Input: dimensioned drawing with shaded views. Units: mm. Origin: part minimum x, y, z. A direction names the side the tool comes from. Coordinates: 2 decimals unless noted, no trailing zeros. Loops run counter-clockwise (first coordinate to the right, second up) from the corner with the lowest first, then second, coordinate; pieces in that order, holes last.
Item 1: Section B-B on x = 49.5. Return loops of the section in (y, z).
Item 2: Contact query for flat-ended pins moving along their axis: P1, Ø12, axis at y = 18, z = 17.5, coming from the -X side; P2, Ø4, axis at x = 32.5, y = 26, coming from the +Z side; P3, Ø6, axis at x = 21.5, y = 37, coming from the +Z side; P4, Ø1, axis at y = 39.5, z = 49.5, coming from the +X side. Output: stop coordinate, or through.
Item 3: Section D-D on z = 40. Return loops of the section in (x, y), and give its area (3 significant figures).
Item 4: Ray query, line 1 along Z through (x, y) = (5.5, 25); line 2 along X through (y, z) = (33, 19); line 3 along Z through (x, y) = (39, 38.5). Return the intervals inside material, ascending.
Item 5: Section A-A on z = 56. Return loops of the section in (x, y), and give its area (3 significant figures).
Item 6: Pull-direction query (Z, two-part tool) for the marked faces 4, 5, 6 and 7; classes: released by +Z, released by -Z, zero draft, split by the parting line, or undercut.
Item 7: Reachability of the marked faces 1, 2 and 3 from +Z, -Z, +X, -X, +Y, -Y: full face, straight path, thin tool, end or side. Return the list, or none.
Item 8: Section C-C on y = 21. Return loops of the section in (x, z).
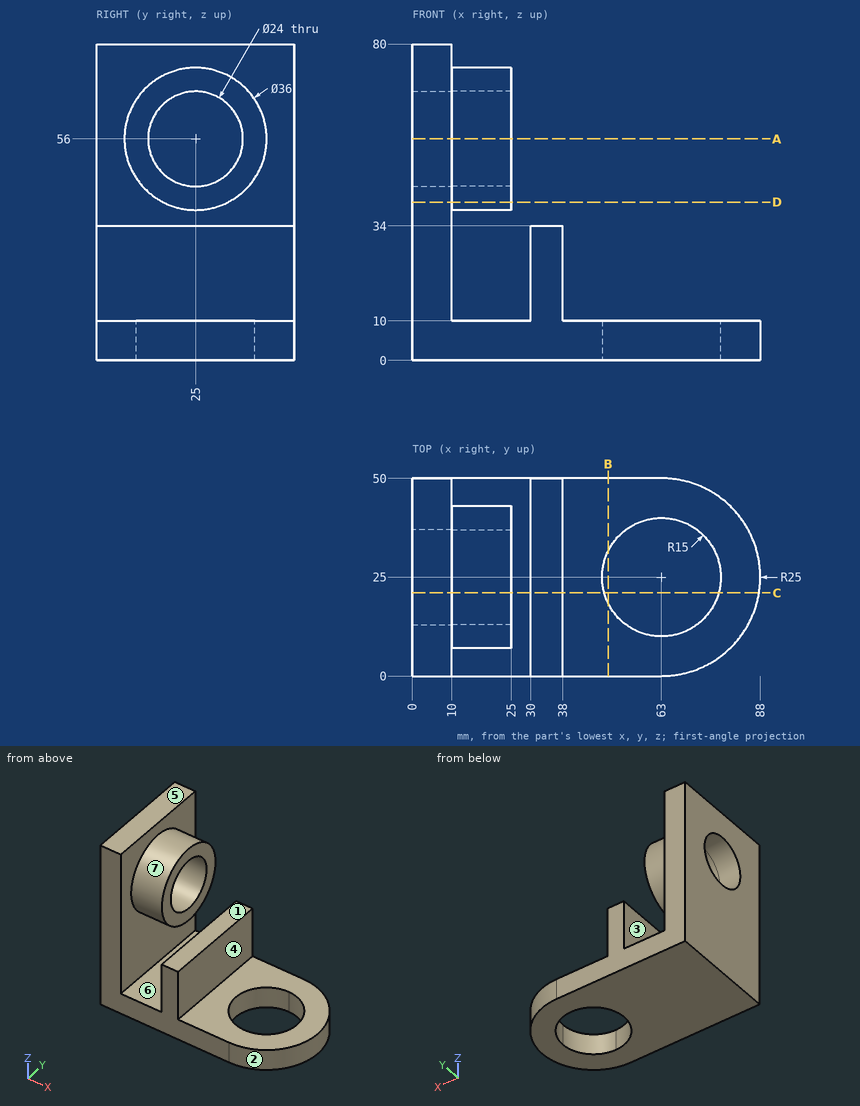
Results found:
1. outline: (0, 0) - (18.46, 0) - (18.46, 10) - (0, 10) - close; (31.54, 0) - (50, 0) - (50, 10) - (31.54, 10) - close
2. P1: stops at x = 0
2. P2: stops at z = 34
2. P3: stops at z = 71.59
2. P4: stops at x = 25
3. outline: (0, 0) - (10, 0) - (10, 16.75) - (25, 16.75) - (25, 33.25) - (10, 33.25) - (10, 50) - (0, 50) - close
3. area: 747 mm2
4. line 1: z = 0 to 44, 68 to 80
4. line 2: x = 0 to 10, 30 to 38
4. line 3: z = 0 to 10
5. outline: (0, 0) - (10, 0) - (10, 7) - (25, 7) - (25, 13) - (0, 13) - close; (0, 37) - (25, 37) - (25, 43) - (10, 43) - (10, 50) - (0, 50) - close
5. area: 440 mm2
6. face 4: zero draft
6. face 5: released by +Z
6. face 6: undercut
6. face 7: undercut
7. face 1: +Z, +X, +Y, -Y
7. face 2: +Z, -Z, +X
7. face 3: +Z, +Y, -Y
8. outline: (0, 0) - (48.54, 0) - (48.54, 10) - (38, 10) - (38, 34) - (30, 34) - (30, 10) - (10, 10) - (10, 38.45) - (25, 38.45) - (25, 44.69) - (0, 44.69) - close; (0, 67.31) - (25, 67.31) - (25, 73.55) - (10, 73.55) - (10, 80) - (0, 80) - close; (77.46, 0) - (87.68, 0) - (87.68, 10) - (77.46, 10) - close
